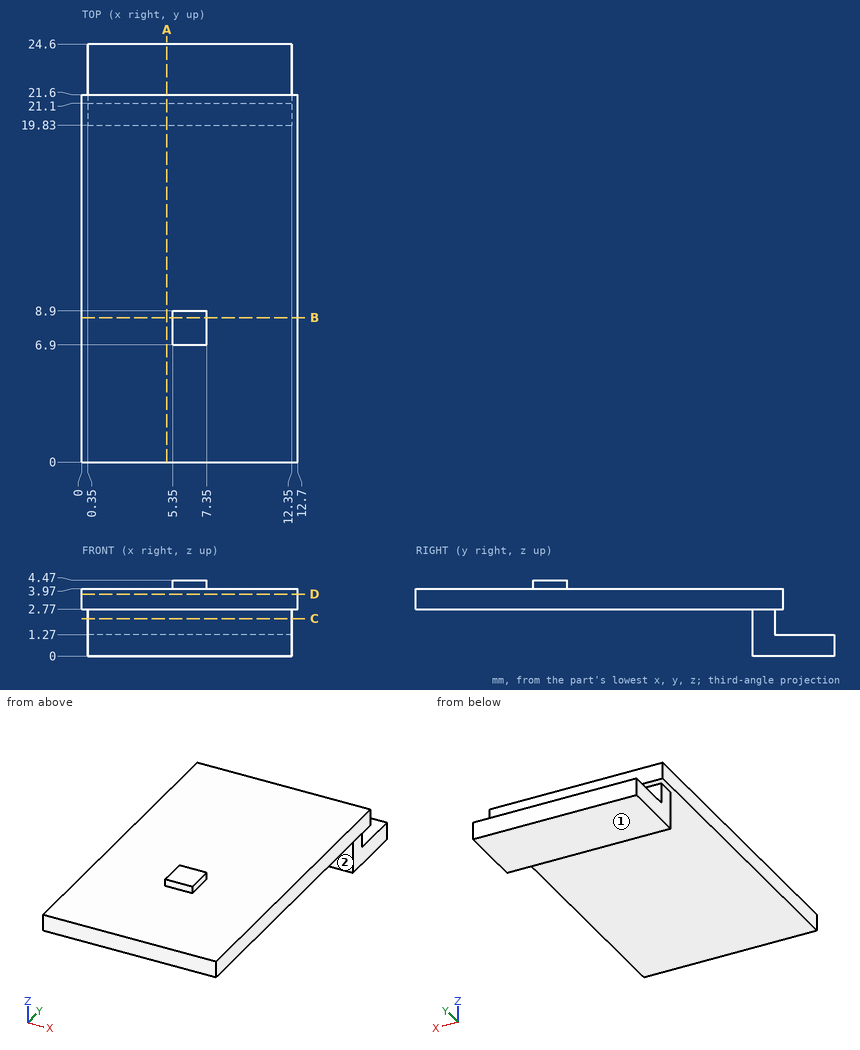
Answer from the drawing. Dimensions are ordinates in mm from the lowest x, y and z of the part. A direction names the side the tool comes from. Coordinates: 2 decimals unless noted, no trailing zeros. Write each loop counter-clockwise with the first axis right and the second up, starting at its lowest first coordinate (ties: lowest second). Pieces come first, ordered by that corner, then holes. Notation, with made-up numbers: M 79,47 L 131,47 A32 ccw 131,77 Z; hole C 60.5,79 d7. An arc over 180 degrees is marked long. Put each result on its own line as item: value. Start each with the question number.
1. A cutting plane is placed at A-A on x = 5. Write down the section's boundary in (y, z).
2. A cutting plane is placed at B-B on y = 8.5. Write down the section's boundary in (x, z).
3. A cutting plane is placed at D-D on z = 3.65. Write down the section's boundary in (x, y), then the cut area to 3 significant figures.
4. Flat-ended cylindrical pins translate along their axes: P1, Ø2, axis at y = 21.5, z = 1, coming from the +X side; P2, Ø0.6, axis at y = 8, z = 4.5, coming from the +X side; P3, Ø1, axis at x = 5, z = 3.5, coming from the +Y side; P4, Ø1.5, axis at x = 6, z = 3.5, coming from the -Y side. Find the tip coordinate at first contact, or state that the pin passes through.
5. A cutting plane is placed at C-C on z = 2.2. Write down the section's boundary in (x, y).
6. Consider line 1 (Y direction, x = 9.5, z = 2.1); line 2 (Y direction, x = 5, z = 2.9); line 3 (Z direction, x = 7.5, y = 7.25). Determine where each line is inside the solid, lowest interval first. Write a range as from..to.
7. Which of the six approach directions +Z, -Z, +X, -X, +Y, -Y give full straight-line access (tool end or side, diameter ignored) to the marked faces 1 and 2?
Resolved:
1. outline: M 0,2.77 L 19.83,2.77 L 19.83,0 L 24.6,0 L 24.6,1.27 L 21.1,1.27 L 21.1,2.77 L 21.6,2.77 L 21.6,3.97 L 0,3.97 Z
2. outline: M 0,2.77 L 12.7,2.77 L 12.7,3.97 L 7.35,3.97 L 7.35,4.47 L 5.35,4.47 L 5.35,3.97 L 0,3.97 Z
3. outline: M 0,0 L 12.7,0 L 12.7,21.6 L 0,21.6 Z
3. area: 274 mm2
4. P1: stops at x = 12.35
4. P2: stops at x = 7.35
4. P3: stops at y = 21.6
4. P4: stops at y = 0
5. outline: M 0.35,19.83 L 12.35,19.83 L 12.35,21.1 L 0.35,21.1 Z
6. line 1: y = 19.83..21.1
6. line 2: y = 0..21.6
6. line 3: z = 2.77..3.97
7. face 1: -Z, +X, -X, +Y, -Y
7. face 2: -Z, +X, -X, -Y
